```python
from build123d import *

# Parameters (mm, degrees)
F1_DEPTH = 127
F2_R     = 6.35
F3_R     = 3.175
F4_R     = 3.175
F5_DEPTH = 6.351
F7_DEPTH = 38.101


with BuildPart() as f1:
    # F0 (on Right) → F1 (new body, symmetric)
    with BuildSketch(Plane.YZ):
        Polygon((-38.1, 0), (0, 0), (0, 38.1), (-6.35, 38.1), (-6.35, 6.35), (-38.1, 6.35), align=None)
    extrude(amount=F1_DEPTH, both=True)

    # F2
    f2_edges = [f1.edges().sort_by_distance(p)[0] for p in [
        (0, -6.35, 6.35),
    ]]
    fillet(f2_edges, radius=F2_R)

    # F3
    f3_edges = [f1.edges().sort_by_distance(p)[0] for p in [
        (0, -6.35, 38.1),
        (0, -38.1, 6.35),
    ]]
    fillet(f3_edges, radius=F3_R)

    # F4 (on face) → F5 (cut, through all)
    with BuildSketch(Plane.XY.offset(6.35)):
        with Locations((-76.2, -23.8125)):
            Circle(F4_R)
        with Locations((76.2, -23.8125)):
            Circle(F4_R)
    extrude(amount=-F5_DEPTH, mode=Mode.SUBTRACT)

    # F6 (on face) → F7 (cut, through all)
    with BuildSketch(Plane(origin=(0, 0, 0), x_dir=(1, 0, 0), z_dir=(0, 0, -1))):
        Polygon((-111.218463, 0), (-127, 38.1), (-127, 0), align=None)
        Polygon((111.218463, 0), (127, 0), (127, 38.1), align=None)
    extrude(amount=-F7_DEPTH, mode=Mode.SUBTRACT)


solid = f1.part
```
Source: CAD feature listing. Evaluate the final solid. Frame: model axes, mm. A direction names the side the tool comes from. Round coordinates to 2 decimals unless told otherwise and drop trailing zeros. Order: outer loops, then holes, each group sorted by start corner. A loop starts at its lowest first (then second) coordinate and runs counter-clockwise, first axis right, second up. Notation, with made-up numbers: (65.25, 31.5) -> (82.25, 31.5) arc R14 ccw to (82.25, 54.5) -> close; hole circle Ø9 at (69, -7.75). An arc over 180 degrees is marked (long way). One line per item, written item: value. Start each with the question number.
Q1. Pin query (flat end, axial travel): pin 1 (6.5 mm diameter, centred on x = 26, y = -29.5, fed in from +Z); pin 2 (2 mm diameter, centred on y = -27.5, z = 4.5, fed in from +X); pin 3 (12 mm diameter, centred on x = 29.5, y = -23, fed in from +Z). Return the tip coordinate at first contact, or that it passes through.
Q2. Section query B-B (x = 12.5). Return the cut outline in (y, z) (3 decimals), plus the area to 3 significant figures.
Q3. Access query for faces 1 (the flat face through (-115.492, -10.317, 6.083)), 2 (the flat face through (2, -24, 6.35)). Directions: +Z, -Z, +X, -X, +Y, -Y. A direction counts if a zero-diameter tool reaches every point of the face in a straight line with its end or side. Return the directions, or none.
Q4. Draft query along X for faces 3 (the flat face through (2, -6.35, 24)), 4 (the cylindrical face through (73.68, -25.744, 3.219)), 5 (the cylindrical face through (-73.17, -22.86, 3.22)), 6 (the flat face through (115.64, -10.67, 6.26)). Return one class per face: pulls with the +X half, pulls with the -X half, needs draft (parallel to the pull), parting line crosses it, or undercut.
Q5. Material intervals for probe 1 along Y at (x, z) = (76, 3); probe 2 along X at (y, z) = (-22, 2); probe 3 along Z at (x, y) = (-82, -3.5), sorted ascending.
Q6. Section query C-C (z = 15). Return the cut outline in (x, y), plus the area to 3 significant figures.
Findings below:
1. pin 1: z = 6.35
1. pin 2: x = 123.02
1. pin 3: z = 6.35
2. outline: (-38.1, 0) -> (0, 0) -> (0, 38.1) -> (-3.175, 38.1) arc R3.175 ccw to (-6.35, 34.925) -> (-6.35, 12.7) arc R6.35 cw to (-12.7, 6.35) -> (-34.925, 6.35) arc R3.175 ccw to (-38.1, 3.175) -> close
2. area: 448 mm²
3. face 1: +Z, -Z, -X, +Y
3. face 2: +Z, +X, -X, -Y
4. face 3: needs draft
4. face 4: undercut
4. face 5: undercut
4. face 6: pulls with the +X half
5. probe 1: -38.1 to -26.98, -20.64 to 0
5. probe 2: -120.33 to -78.81, -73.59 to 73.59, 78.81 to 120.33
5. probe 3: 0 to 38.08
6. outline: (-113.85, -6.35) -> (113.85, -6.35) -> (111.22, 0) -> (-111.22, 0) -> close
6. area: 1,430 mm²
